Model file for the job. Use its own axes, mm. Face numbers are marked on the shaded views. Round coordinates to 2 decimals unless told otherwise and drop trailing zeros. Order: outer loops, then holes, each group sorted by start corner. A loop starts at its lowest first (then second) coordinate and runs counter-clockwise, first axis right, second up. Notation, with made-up numbers: M 61,76 L 91,76 A9 cw 91,82 Z; hole C 29.25,51 d2. An arc over 180 degrees is marked long. Return JSON: item names as keys, results as strings. Group by question number.
Item 1: Slice it at A-A on z = 0.75. Write the cut outline in (x, y).
Item 2: Probe line 1 along X through (y, z) = (275, -6.3); line 2 along Z through (x, y) = (5, 100.5). List the from-to ranges inside material, lowest first.
Item 3: Slice it at C-C on x = -1. Give the number of separate pieces and of enclosed holes in the cut face, then the cut area to 3 significant figures.
Item 4: Pull direction X, two halves, no side cores. Call the marked faces 1, 2 and 3: pulls with the +X half, pulls with the -X half, needs draft (parallel to the pull), parting line crosses it, or undercut.
Item 5: Slice it at B-B on y = 5. Write the cut outline in (x, z), then the cut area to 3 significant figures.
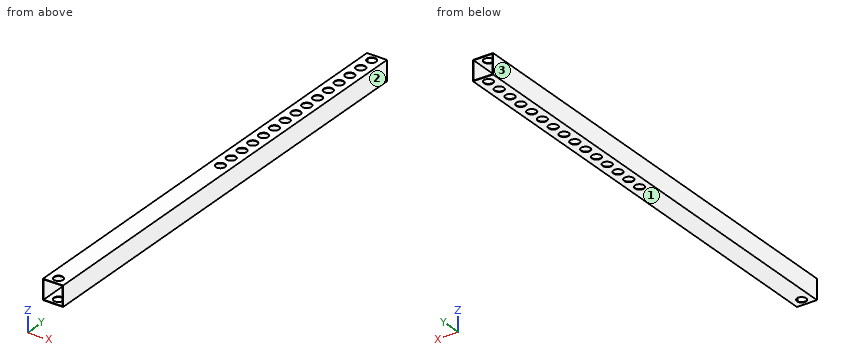
from build123d import *

# Parameters (mm, degrees)
CROQUIS1_W              = 13
CROQUIS1_H              = 13
SALIENTE_EXTRUIR1_DEPTH = 300
CROQUIS2_W              = 12.366
CROQUIS2_H              = 12.366
CORTAR_EXTRUIR1_DEPTH   = 500
CROQUIS3_R              = 3
CORTAR_EXTRUIR2_DEPTH   = 500
CROQUIS4_R              = 3
CORTAR_EXTRUIR3_DEPTH   = 500


with BuildPart() as part:
    # Croquis1 → Saliente-Extruir1 (new body)
    with BuildSketch(Plane(origin=(0, 0, 0), x_dir=(1, 0, 0), z_dir=(0, 1, 0))):
        Rectangle(CROQUIS1_W, CROQUIS1_H)
    extrude(amount=SALIENTE_EXTRUIR1_DEPTH)

    # Croquis2 → Cortar-Extruir1 (cut)
    with BuildSketch(Plane(origin=(0, 300, 0), x_dir=(1, 0, 0), z_dir=(0, 1, 0))):
        Rectangle(CROQUIS2_W, CROQUIS2_H)
    extrude(amount=-CORTAR_EXTRUIR1_DEPTH, mode=Mode.SUBTRACT)

    # Croquis3 → Cortar-Extruir2 (cut)
    with BuildSketch(Plane.XY.offset(6.5)):
        with Locations((0, 5)):
            Circle(CROQUIS3_R)
    extrude(amount=-CORTAR_EXTRUIR2_DEPTH, mode=Mode.SUBTRACT)

    # Croquis4 → Cortar-Extruir3 (cut)
    with BuildSketch(Plane.XY.offset(6.5)):
        with Locations((0, 295)):
            Circle(CROQUIS4_R)
        with Locations((0, 285)):
            Circle(CROQUIS4_R)
        with Locations((0, 275)):
            Circle(CROQUIS4_R)
        with Locations((0, 265)):
            Circle(CROQUIS4_R)
        with Locations((0, 255)):
            Circle(CROQUIS4_R)
        with Locations((0, 245)):
            Circle(CROQUIS4_R)
        with Locations((0, 235)):
            Circle(CROQUIS4_R)
        with Locations((0, 225)):
            Circle(CROQUIS4_R)
        with Locations((0, 215)):
            Circle(CROQUIS4_R)
        with Locations((0, 205)):
            Circle(CROQUIS4_R)
        with Locations((0, 195)):
            Circle(CROQUIS4_R)
        with Locations((0, 185)):
            Circle(CROQUIS4_R)
        with Locations((0, 175)):
            Circle(CROQUIS4_R)
        with Locations((0, 165)):
            Circle(CROQUIS4_R)
        with Locations((0, 155)):
            Circle(CROQUIS4_R)
    extrude(amount=-CORTAR_EXTRUIR3_DEPTH, mode=Mode.SUBTRACT)


solid = part.part
Output values:
{
 "1": {"outline": "M -6.5,0 L -6.18,0 L -6.18,300 L -6.5,300 Z; M 6.18,0 L 6.5,0 L 6.5,300 L 6.18,300 Z"},
 "2": {"line 1": "-6.5 to -3, 3 to 6.5", "line 2": "-6.5 to -6.18, 6.18 to 6.5"},
 "3": {"separate pieces": "34", "enclosed holes": "0", "area": "133 mm²"},
 "4": {"face 1": "needs draft", "face 2": "pulls with the +X half", "face 3": "pulls with the -X half"},
 "5": {"outline": "M -6.5,-6.5 L -3,-6.5 L -3,-6.18 L -6.18,-6.18 L -6.18,6.18 L -3,6.18 L -3,6.5 L -6.5,6.5 Z; M 3,-6.5 L 6.5,-6.5 L 6.5,6.5 L 3,6.5 L 3,6.18 L 6.18,6.18 L 6.18,-6.18 L 3,-6.18 Z", "area": "12.3 mm²"}
}
